Verification items for the finished model (mm, model axes). Face numbers are marked on the shaded views. A direction names the side the tool comes from. Coordinates: 2 decimals unless noted, no trailing zeros. Order: outer loops, then holes, each group sorted by start corner. A loop starts at its lowest first (then second) coordinate and runs counter-clockwise, first axis right, second up. Notation, with made-up numbers: (69.25, 31) -> (111.25, 31) arc R15 ccw to (111.25, 43) -> close; hole circle Ø3 at (42, 11). An arc over 180 degrees is marked (long way). Write item = value, one per line. Start each with the question number.
1. Cross-section at A-A on y = -0.75. Record the cut outline in (x, z), plus the area to 3 significant figures.
2. Cross-section at C-C on x = 1. Record the cut outline in (y, z).
3. Go/stop test with flat-tipped pins: P1, Ø5, axis at y = -5.5, z = 4, coming from the -X side; P2, Ø10, axis at x = -4, y = -13.5, coming from the -Z side; P3, Ø4, axis at y = -14, z = 9, coming from the +X side; P4, Ø7, axis at x = -4.5, z = 9, coming from the -Y side. Record where each tip stops, or that it passes through.
4. Cross-section at D-D on y = -7.25. Record the cut outline in (x, z), plus the area to 3 significant figures.
5. Cross-section at B-B on z = 1.75. Record the cut outline in (x, y), plus the area to 3 significant figures.
6. Thickness scan on line 1 along Y through (x, z) = (10, 4.25); line 2 along X through (y, z) = (-0.5, 6); line 3 along X through (y, z) = (-12.75, 11). Record the ranges inside material, lowest first. Write a range as from..to.
7. Set-up check for the marked faces 1 and 2: record each of +Z, -Z, +X, -X, +Y, -Y from which the full face is reachable in a straight line by a thin tool's end or side.
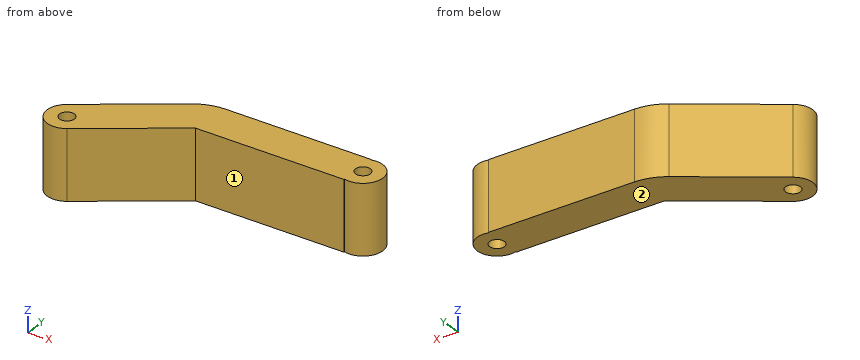
from build123d import *

# Parameters (mm, degrees)
SKETCH_1_R      = 1.5
EXTRUDE_2_DEPTH = 14
FILLET_1_R      = 10


with BuildPart() as part:
    # 草图1 → 凸台-拉伸2 (new body)
    with BuildSketch(Plane.XY):
        with BuildLine():
            Line((15.60515688, 4.016530447), (15.60515688, 4.161375168))
            Line((15.60515688, 4.161375168), (-16.917233431, 4.161375168))
            Line((-16.917233431, 4.161375168), (-36.422020871, -9.496024029))
            ThreePointArc((-36.422020871, -9.496024029), (-37.404323302, -15.066937951), (-31.83340938, -16.049240383))
            Line((-31.83340938, -16.049240383), (-14.39484312, -3.838624832))
            Line((-14.39484312, -3.838624832), (15.60515688, -3.838624832))
            Line((15.60515688, -3.838624832), (15.60515688, -3.693780111))
            ThreePointArc((15.60515688, -3.693780111), (20.671823547, 0.161375168), (15.60515688, 4.016530447))
        make_face()
        with Locations((-34.127715125, -12.772632206)):
            Circle(SKETCH_1_R, mode=Mode.SUBTRACT)
        with Locations((16.671823547, 0.161375168)):
            Circle(SKETCH_1_R, mode=Mode.SUBTRACT)
    extrude(amount=EXTRUDE_2_DEPTH)

    # 圆角1
    fillet_1_edges = [part.edges().sort_by_distance(p)[0] for p in [
        (-16.917233431, 4.161375168, 7),
    ]]
    fillet(fillet_1_edges, radius=FILLET_1_R)


solid = part.part
Worked out:
q1.outline = (-23.93, 0) -> (15.48, 0) -> (15.48, 14) -> (-23.93, 14) -> close; (17.86, 0) -> (20.57, 0) -> (20.57, 14) -> (17.86, 14) -> close
q1.area = 590 mm²
q2.outline = (-3.84, 0) -> (4.16, 0) -> (4.16, 14) -> (-3.84, 14) -> close
q3.P1 = -34.29
q3.P2 = through
q3.P3 = -26.05
q3.P4 = -3.84
q4.outline = (-33.21, 0) -> (-19.27, 0) -> (-19.27, 14) -> (-33.21, 14) -> close
q4.area = 195 mm²
q5.outline = (-36.42, -9.5) arc R4 ccw to (-31.83, -16.05) -> (-14.39, -3.84) -> (15.61, -3.84) -> (15.61, -3.69) arc R4 ccw (long way) to (15.61, 4.02) -> (15.61, 4.16) -> (-13.76, 4.16) arc R10 ccw to (-19.5, 2.35) -> close; hole circle Ø3 at (-34.13, -12.77); hole circle Ø3 at (16.67, 0.16)
q5.area = 474 mm²
q6.line_1 = -3.84..4.16
q6.line_2 = -23.57..15.33, 18.02..20.62
q6.line_3 = -38.13..-35.63, -32.63..-27.12
q7.face_1 = +Z, -Z, +X, -Y
q7.face_2 = -Z, +X, -X, +Y, -Y
